from build123d import *

# Parameters (mm, degrees)
BOSS_EXTRUDE1_DEPTH = 3.175
SKETCH2_R           = 2
CUT_EXTRUDE1_DEPTH  = 72.912172996
CUT_EXTRUDE2_START  = -3.175
CUT_EXTRUDE2_DEPTH  = 2
BOSS_EXTRUDE2_DEPTH = 3.175


with BuildPart() as part:
    # Sketch1 → Boss-Extrude1 (new body)
    with BuildSketch(Plane(origin=(0, 0, 0), x_dir=(1, 0, 0), z_dir=(0, 1, 0))):
        Polygon((0, 0), (50.8, 0), (0, 50.8), align=None)
    extrude(amount=BOSS_EXTRUDE1_DEPTH)

    # Sketch2 → Cut-Extrude1 (cut, through all)
    with BuildSketch(Plane(origin=(0, 3.175, 0), x_dir=(1, 0, 0), z_dir=(0, 1, 0))):
        with Locations(Location((19.05, 6.35, 0), (0, 0, 270))):
            Circle(SKETCH2_R)
        with Locations(Location((6.35, 19.05, 0), (0, 0, 90))):
            Circle(SKETCH2_R)
    extrude(amount=-CUT_EXTRUDE1_DEPTH, mode=Mode.SUBTRACT)

    # Sketch3 → Cut-Extrude2 (cut)
    with BuildSketch(Plane(origin=(0, 3.175, 0), x_dir=(1, 0, 0), z_dir=(0, 1, 0)).offset(CUT_EXTRUDE2_START)):
        Polygon((8.370723055, 15.550005), (10.391446111, 19.05), (8.370723055, 22.549995), (4.329276945, 22.549995), (2.308553889, 19.05), (4.329276945, 15.550005), align=None)
        Polygon((22.549995, 4.329276945), (19.05, 2.308553889), (15.550005, 4.329276945), (15.550005, 8.370723055), (19.05, 10.391446111), (22.549995, 8.370723055), align=None)
    extrude(amount=CUT_EXTRUDE2_DEPTH, mode=Mode.SUBTRACT)

    # Sketch4 → Boss-Extrude2 (add, through all)
    with BuildSketch(Plane(origin=(0, 0, 0), x_dir=(-1, 0, 0), z_dir=(0, -1, 0))):
        with BuildLine():
            Line((0, 0), (-74.904635469, 0))
            Line((-74.904635469, 0), (-74.904635469, -40))
            Line((-74.904635469, -40), (20.871249235, -40))
            ThreePointArc((20.871249235, -40), (61.323705254, -22.707621637), (78.006543383, 18))
            Line((78.006543383, 18), (78.006543383, 53.511510239))
            Line((78.006543383, 53.511510239), (38, 53.511510239))
            Line((38, 53.511510239), (38, 18))
            ThreePointArc((38, 18), (32.727922061, 5.272077939), (20, 0))
            Line((20, 0), (0, 0))
        make_face()
    extrude(amount=-BOSS_EXTRUDE2_DEPTH)


solid = part.part
Could you check a few things on this model? Use its own coordinates, in mm. A direction names the side the tool comes from. Give positions to 0.01 mm unless a question says otherwise; leave off trailing zeros. Order: outer loops, then holes, each group sorted by start corner. A loop starts at its lowest first (then second) coordinate and runs counter-clockwise, first axis right, second up. Notation, with made-up numbers: (-28, 23.25) -> (-10, 23.25) arc R14 ccw to (-10, 28.25) -> close; hole circle Ø5 at (5.25, 83). An arc over 180 degrees is marked (long way). Return JSON: item names as keys, results as strings.
1. Imagine slicing it at C-C on z = -36. List the corners of the cut face in (x, y) for me (3 decimals).
Answer list:
{"outline": "(-78.007, 0) -> (-38, 0) -> (-38, 3.175) -> (-78.007, 3.175) -> close; (0, 0) -> (14.8, 0) -> (14.8, 3.175) -> (0, 3.175) -> close"}
2. I need wall thicknesses on line 1 (X direction, y = 2.75, z = -6.35); line 2 (X direction, y = 0.95, z = -6.5); line 3 (Z direction, x = -5, y = 0.3). Which ranges of each line are inside material? Lowest first, please. Write a range as from..to.
Answer list:
{"line 1": "x = -76.82..-33.72, 0..17.05, 21.05..44.45", "line 2": "x = -76.86..-33.85, 0..15.55, 22.55..44.3", "line 3": "z = 0..40"}
3. Imagine slicing it at D-D on z = -6.35. List the corners of the cut face in (x, y) for me (3 decimals), then the cut area to 3 significant figures.
Answer list:
{"outline": "(-76.825, 0) -> (-33.721, 0) -> (-33.721, 3.175) -> (-76.825, 3.175) -> close; (0, 0) -> (15.55, 0) -> (15.55, 2) -> (17.05, 2) -> (17.05, 3.175) -> (0, 3.175) -> close; (21.05, 2) -> (22.55, 2) -> (22.55, 0) -> (44.45, 0) -> (44.45, 3.175) -> (21.05, 3.175) -> close", "area": "259 mm2"}
4. For pin 1 Ø0.6 at (x, y) = (6.5, 1) entering from -Z; pin 2 Ø1.6 at (y, z) = (1, -7) entering from +X; pin 3 Ø3.5 at (x, z) = (6.5, -18.5) entering from -Y, each with a flat end and sliding along its axis, tell me the tip position at first contact or that it passes through.
Answer list:
{"pin 1": "stops at z = -44.6", "pin 2": "stops at x = 44.6", "pin 3": "stops at y = 2"}
5. Thinking about a two-plate mould opening in X: for faces 4 (the flat face through (63, 2, 0)), 5 (the flat face through (25.8, 1.6, -25)), 6 (the flat face through (0, 2, -26)), which applies, pulls with the +X half, pulls with the -X half, needs draft (parallel to the pull), parting line crosses it, or undercut?
Answer list:
{"face 4": "needs draft", "face 5": "pulls with the +X half", "face 6": "undercut"}
6. On a 3-axis mill with a long thin cutter (end or side, diameter ignored), from which of +Z, -Z, +X, -X, +Y, -Y can I reach the whole of each face in a straight line? I mean faces 1 (the cylindrical face through (6.262, 2.596, -17.052)), 2 (the cylindrical face through (-32.867, 1.565, -5.413)), 3 (the flat face through (8, 2, -21)). Say none if no direction works.
Answer list:
{"face 1": "+Y, -Y", "face 2": "-Z, +Y, -Y", "face 3": "-Y"}
7. Imagine slicing it at B-B on x = 6.35. List the corners of the cut face in (y, z) for me (3 decimals), then the cut area to 3 significant figures.
Answer list:
{"outline": "(0, -44.45) -> (3.175, -44.45) -> (3.175, -21.05) -> (2, -21.05) -> (2, -22.55) -> (0, -22.55) -> close; (0, -15.55) -> (2, -15.55) -> (2, -17.05) -> (3.175, -17.05) -> (3.175, 40) -> (0, 40) -> close", "area": "249 mm2"}
8. Imagine slicing it at A-A on y = 0.6. List the corners of the cut face in (x, z) for me.
Answer list:
{"outline": "(-78.01, -53.51) -> (-38, -53.51) -> (-38, -18) arc R18 cw to (-20, 0) -> (0, 0) -> (0, -50.8) -> (50.8, 0) -> (74.9, 0) -> (74.9, 40) -> (-20.87, 40) arc R58.01 ccw to (-78.01, -18) -> close; hole (2.31, -19.05) -> (4.33, -22.55) -> (8.37, -22.55) -> (10.39, -19.05) -> (8.37, -15.55) -> (4.33, -15.55) -> close; hole (15.55, -8.37) -> (19.05, -10.39) -> (22.55, -8.37) -> (22.55, -4.33) -> (19.05, -2.31) -> (15.55, -4.33) -> close"}
